```python
from build123d import *

# Parameters (mm, degrees)
F1_DEPTH  = 20
F2_R      = 2.6
F3_DEPTH  = 19.1431356237
F4_R      = 2.5
F5_DEPTH  = 5.001
F6_R      = 3.05
F7_DEPTH  = 2
F8_W      = 5
F8_H      = 20
F9_DEPTH  = 25
F11_D     = 3
F11_DEPTH = 10
F11_TIP   = 0.9012909285


with BuildPart() as f1:
    # F0 (on Front) → F1 (new body)
    with BuildSketch(Plane.XZ):
        Polygon((-65, 0), (0, 0), (0, 5), (-62.9289321881, 5), (-81.4644660941, 23.5355339059), (-85, 20), align=None)
    extrude(amount=F1_DEPTH)

    # F2 (on face) → F3 (cut, through all)
    with BuildSketch(Plane(origin=(-28.9644660941, 0, -28.9644660941), x_dir=(0.7071067812, 0, -0.7071067812), z_dir=(0.7071067812, 0, 0.7071067812))):
        with Locations((-70.2462120246, -10)):
            Circle(F2_R)
    extrude(amount=-F3_DEPTH, mode=Mode.SUBTRACT)

    # F4 (on face) → F5 (cut, through all)
    with BuildSketch(Plane.XY.offset(5)):
        with Locations((-12.9289321881, -10)):
            Circle(F4_R)
    extrude(amount=-F5_DEPTH, mode=Mode.SUBTRACT)

    # F6 (on face) → F7 (cut)
    with BuildSketch(Plane(origin=(-28.9644660941, 0, -28.9644660941), x_dir=(0.7071067812, 0, -0.7071067812), z_dir=(0.7071067812, 0, 0.7071067812))):
        with Locations((-70.2462120246, -10)):
            Circle(F6_R)
    extrude(amount=-F7_DEPTH, mode=Mode.SUBTRACT)

    # F8 (on face) → F9 (join)
    with BuildSketch(Plane.XY.offset(5)):
        with Locations((-2.5, -10)):
            Rectangle(F8_W, F8_H)
    extrude(amount=F9_DEPTH)

    # F11
    with Locations(Plane.XY.offset(30)):
        with Locations((-2.5, -16), (-2.5, -4)):
            Hole(F11_D / 2, depth=F11_DEPTH)
            with Locations((0, 0, -(F11_DEPTH + F11_TIP / 2))):  # 118° drill point
                Cone(0, F11_D / 2, F11_TIP, mode=Mode.SUBTRACT)


solid = f1.part
```
Build history of the part. All positions in model axes, mm. A direction names the side the tool comes from. Round coordinates to 2 decimals unless told otherwise and drop trailing zeros. Loops run counter-clockwise (first coordinate to the right, second up) from the corner with the lowest first, then second, coordinate; pieces in that order, holes last.
Item 1: Saw through at D-D (z = 3.5). List the corners of the cut face in (x, y).
Item 2: Which spindle directions (+Z, -Z, +X, -X, +Y, -Y) get a long thin tool onto all of the face, cutting with end or side? Do faces 5 (the face through (-5, -10, 17)), 6 (the face through (-13.47, -12.44, 2.54)), 7 (the face through (-2.175, -17.464, 24.93)). Say none if no direction does.
Item 3: Saw through at B-B (y = -1.5). List the corners of the cut face in (x, z).
Item 4: Pin check, flat tips, straight feed: P1, Ø4, axis at x = -12.93, y = -10, coming from the +Z side; P2, Ø10, axis at x = -23.5, y = -6.5, coming from the +Z side; P3, Ø2, axis at x = -68, y = -5, coming from the -Z side. Stop position of each tip, or through.
Item 5: Two-plate mould, pull along Z, no slides. Class faces 1 (the face through (-72.07, -9.86, 14.14)), 2 (the face through (-36, 0, 4)), 3 (the face through (-80.25, -12.31, 17.4)), 4 (the face through (-77.28, -9.08, 17.95)): released by +Z, released by -Z, zero draft, split by the parting line, or undercut.
Item 6: Drill centre lines: line 1 along Y through (x, z) = (-2.5, 23.75); line 2 along X through (y, z) = (-16, 26); line 3 along X through (y, z) = (-15.75, 19.5). Where is each one in solid material? Low to high.
Item 7: Saw through at A-A (z = 13). List the corners of the cut face in (x, y).
Item 8: Saw through at C-C (z = 28.5). List the corners of the cut face in (x, y), then the cut area to 3 significant figures.
Worked answers:
1. outline: (-68.5, -20) - (0, -20) - (0, 0) - (-68.5, 0) - close; hole circle Ø5 at (-12.93, -10)
2. face 5: +Z, +Y, -Y
2. face 6: +Z, -Z
2. face 7: +Z
3. outline: (-85, 20) - (-65, 0) - (0, 0) - (0, 30) - (-5, 30) - (-5, 5) - (-62.93, 5) - (-81.46, 23.54) - close
4. P1: passes through
4. P2: stops at z = 5
4. P3: stops at z = 2
5. face 1: released by +Z
5. face 2: zero draft
5. face 3: undercut
5. face 4: undercut
6. line 1: y = -20 to -17.5, -14.5 to -5.5, -2.5 to 0
6. line 2: x = -5 to -4, -1 to 0
6. line 3: x = -84.5 to -77.43, -5 to -3.12, -1.88 to 0
7. outline: (-78, -20) - (-70.93, -20) - (-70.93, 0) - (-78, 0) - close; (-5, -20) - (0, -20) - (0, 0) - (-5, 0) - close
8. outline: (-5, -20) - (0, -20) - (0, 0) - (-5, 0) - close; hole circle Ø3 at (-2.5, -16); hole circle Ø3 at (-2.5, -4)
8. area: 85.9 mm2
